from build123d import *

# Parameters (mm, degrees)
SKETCH1_W                    = 93
SKETCH1_H                    = 20
BOSS_EXTRUDE1_DEPTH          = 6
CUT_EXTRUDE1_REACH           = 49.94
SKETCH2_W                    = 73
SKETCH2_H                    = 9
F_6_0_204_DIAMETER_HOLE1_D   = 5.1816
F_6_CLEARANCE_HOLE1_D        = 3.7973
F_6_32_TAPPED_HOLE1_REACH    = 52.973
F_6_32_TAPPED_HOLE1_BORE_R   = 1.35255
F_1_8_0_125_DIAMETER_HOLE1_D = 3.175
FILLET1_R                    = 1
CHAMFER1_SIZE                = 0.5


with BuildPart() as part:
    # Sketch1 → Boss-Extrude1 (new body)
    with BuildSketch(Plane.XY):
        Rectangle(SKETCH1_W, SKETCH1_H)
    extrude(amount=BOSS_EXTRUDE1_DEPTH)

    # Sketch2 → Cut-Extrude1 (cut, up to next)
    with BuildSketch(Plane.XY.offset(6), mode=Mode.PRIVATE) as cut_extrude1_sk1:
        with Locations((0, -5.5)):
            Rectangle(SKETCH2_W, SKETCH2_H)
    cut_extrude1_tool1 = extrude(cut_extrude1_sk1.sketch, amount=-CUT_EXTRUDE1_REACH, mode=Mode.PRIVATE) & part.part
    add(cut_extrude1_tool1.solids().sort_by_distance((0, -5.5, 6))[0], mode=Mode.SUBTRACT)

    # #6 (0.204) Diameter Hole1 (through all)
    with Locations(Plane.XY.offset(6)):
        with Locations((42, -4), (-42, -4)):
            Hole(F_6_0_204_DIAMETER_HOLE1_D / 2)

    # #6 Clearance Hole1 (through all)
    with Locations(Plane(origin=(0, 10, 0), x_dir=(1, 0, 0), z_dir=(0, 1, 0))):
        with Locations((18, -3)):
            Hole(F_6_CLEARANCE_HOLE1_D / 2)

    # #6-32 Tapped Hole1 bore → #6-32 Tapped Hole1 (cut, up to next)
    with BuildSketch(Plane(origin=(0, 10, 0), x_dir=(1, 0, 0), z_dir=(0, 1, 0)), mode=Mode.PRIVATE) as f_6_32_tapped_hole1_sk1:
        with Locations((-42, -3)):
            Circle(F_6_32_TAPPED_HOLE1_BORE_R)
    f_6_32_tapped_hole1_tool1 = extrude(f_6_32_tapped_hole1_sk1.sketch, amount=-F_6_32_TAPPED_HOLE1_REACH, mode=Mode.PRIVATE) & part.part
    # #6-32 Tapped Hole1 bore → #6-32 Tapped Hole1 (cut, up to next)
    with BuildSketch(Plane(origin=(0, 10, 0), x_dir=(1, 0, 0), z_dir=(0, 1, 0)), mode=Mode.PRIVATE) as f_6_32_tapped_hole1_sk2:
        with Locations((42, -3)):
            Circle(F_6_32_TAPPED_HOLE1_BORE_R)
    f_6_32_tapped_hole1_tool2 = extrude(f_6_32_tapped_hole1_sk2.sketch, amount=-F_6_32_TAPPED_HOLE1_REACH, mode=Mode.PRIVATE) & part.part
    add(f_6_32_tapped_hole1_tool1.solids().sort_by_distance((-42, 10, 3))[0], mode=Mode.SUBTRACT)
    add(f_6_32_tapped_hole1_tool2.solids().sort_by_distance((42, 10, 3))[0], mode=Mode.SUBTRACT)

    # 1/8 (0.125) Diameter Hole1 (through all)
    with Locations(Plane(origin=(0, 10, 0), x_dir=(1, 0, 0), z_dir=(0, 1, 0))):
        with Locations((-18, -3)):
            Hole(F_1_8_0_125_DIAMETER_HOLE1_D / 2)

    # Fillet1
    fillet1_edges = [part.edges().sort_by_distance(p)[0] for p in [
        (-36.5, -10, 3),
        (-36.5, -1, 3),
        (36.5, -1, 3),
        (36.5, -10, 3),
        (46.5, -10, 3),
        (-46.5, -10, 3),
        (-46.5, 10, 3),
        (46.5, 10, 3),
    ]]
    fillet(fillet1_edges, radius=FILLET1_R)

    # Chamfer1
    chamfer1_edges = [part.edges().sort_by_distance(p)[0] for p in [
        (44.5908, -4, 6),
        (44.5908, -4, 0),
        (-39.4092, -4, 6),
        (-39.4092, -4, 0),
        (19.89865, 10, 3),
        (19.89865, -1, 3),
        (40.64745, 10, 3),
        (-43.35255, 10, 3),
        (-16.4125, 10, 3),
        (-16.4125, -1, 3),
    ]]
    chamfer(chamfer1_edges, length=CHAMFER1_SIZE)


solid = part.part
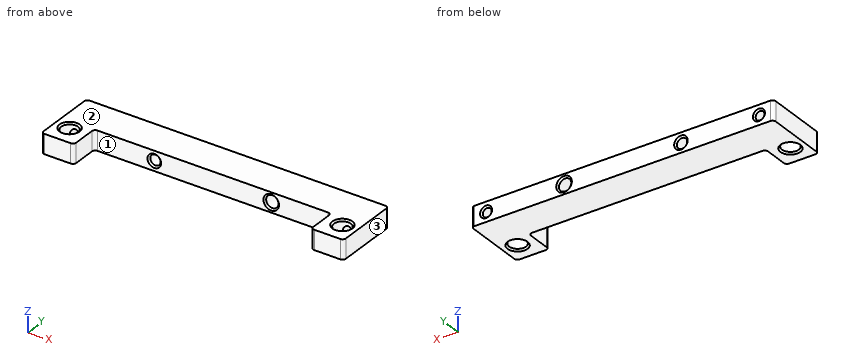
Design review of the part built by this model. Coordinates are the model's own, in mm. Face numbers are marked on the shaded views. Coordinates: 2 decimals unless noted, no trailing zeros. Loops run counter-clockwise (first coordinate to the right, second up) from the corner with the lowest first, then second, coordinate; pieces in that order, holes last.
Item 1: Add section A-A (y = 3). Write out the cut boundary in (x, z) (1 decimal), and give its area (3 significant figures).
Completed:
outline: (-46.5, 0) - (46.5, 0) - (46.5, 6) - (-46.5, 6) - close; hole circle Ø2.7 at (-42, 3); hole circle Ø3.2 at (-18, 3); hole circle Ø3.8 at (18, 3); hole circle Ø2.7 at (42, 3)
area: 527 mm2
Item 2: Clearance check with flat-ended pins moving along their axes: pin 1 (6 mm diameter, centred on x = 42, y = -4, fed in from +Z); pin 2 (2.5 mm diameter, centred on x = 18, z = 3, fed in from -Y); pin 3 (8 mm diameter, centred on x = -13.5, y = -1.5, fed in from +Z); pin 4 (3 mm diameter, centred on x = 42, z = 3, fed in from +Y). State where each tip first meets the part, or that it passes through.
Completed:
pin 1: stops at z = 5.91
pin 2: passes through
pin 3: stops at z = 6
pin 4: stops at y = 9.65
Item 3: Draft analysis for pull direction X (two halves, no side actions). For the marked faces 1, 2 and 3, state which applies: pulls with the +X half, pulls with the -X half, needs draft (parallel to the pull), parting line crosses it, or undercut.
Completed:
face 1: undercut
face 2: needs draft
face 3: pulls with the +X half
Item 4: Add section D-D (x = 18). Write out the cut boundary in (y, z), and give its area (3 significant figures).
Completed:
outline: (-1, 0) - (10, 0) - (10, 0.6) - (9.5, 1.1) - (-0.5, 1.1) - (-1, 0.6) - close; (-1, 5.4) - (-0.5, 4.9) - (9.5, 4.9) - (10, 5.4) - (10, 6) - (-1, 6) - close
area: 23.7 mm2
Item 5: Add section B-B (x = -42). Write out the cut boundary in (y, z), and give its area (3 significant figures).
Completed:
outline: (-10, 0) - (-7.09, 0) - (-6.59, 0.5) - (-6.59, 5.5) - (-7.09, 6) - (-10, 6) - close; (-1.41, 0.5) - (-0.91, 0) - (10, 0) - (10, 1.15) - (9.5, 1.65) - (-1.41, 1.65) - close; (-1.41, 4.35) - (9.5, 4.35) - (10, 4.85) - (10, 6) - (-0.91, 6) - (-1.41, 5.5) - close
area: 57.3 mm2
Item 6: Add section C-C (y = -4). Write out the cut boundary in (x, z), and give its area (3 significant figures).
Completed:
outline: (-46.5, 0) - (-45.09, 0) - (-44.59, 0.5) - (-44.59, 5.5) - (-45.09, 6) - (-46.5, 6) - close; (-39.41, 0.5) - (-38.91, 0) - (-36.5, 0) - (-36.5, 6) - (-38.91, 6) - (-39.41, 5.5) - close; (36.5, 0) - (38.91, 0) - (39.41, 0.5) - (39.41, 5.5) - (38.91, 6) - (36.5, 6) - close; (44.59, 0.5) - (45.09, 0) - (46.5, 0) - (46.5, 6) - (45.09, 6) - (44.59, 5.5) - close
area: 56.8 mm2
Item 7: Wall thickness on L1, parallel to X at y = 2, z = 3; L2, parallel to X at y = -2.75, z = 5.3; L3, parallel to Z at x = -42, y = 5.25: over which ranges is each line inside the solid? List them lowest first.
Completed:
L1: x = -46.5 to -43.35, -40.65 to -19.59, -16.41 to 16.1, 19.9 to 40.65, 43.35 to 46.5
L2: x = -46.5 to -44.27, -39.73 to -36.5, 36.5 to 39.73, 44.27 to 46.5
L3: z = 0 to 1.65, 4.35 to 6
